from build123d import *

# Parameters (mm, degrees)
SKETCH1_R           = 1.375
BOSS_EXTRUDE1_DEPTH = 1.19
CHAMFER1_SIZE       = 0.25


with BuildPart() as part:
    # Sketch1 → Boss-Extrude1 (new, symmetric)
    with BuildSketch(Plane(origin=(0, 0, 0), x_dir=(1, 0, 0), z_dir=(0, 1, 0))):
        Polygon((0, 3.175426481), (-2.75, 1.58771324), (-2.75, -1.58771324), (0, -3.175426481), (2.75, -1.58771324), (2.75, 1.58771324), align=None)
        with Locations(Location((0, 0, 0), (0, 0, 270))):
            Circle(SKETCH1_R, mode=Mode.SUBTRACT)
    extrude(amount=BOSS_EXTRUDE1_DEPTH, both=True)

    # Sketch2 → Cut-Revolve1 (revolve, cut)
    with BuildSketch(Plane(origin=(0, 0, 0), x_dir=(0, 0, -1), z_dir=(1, 0, 0))):
        Polygon((2.7, 1.19), (3.175426481, 0.89), (3.175426481, 1.19), align=None)
    cut_revolve1 = revolve(axis=Axis((0, 0, 0), (0, 1, 0)), mode=Mode.SUBTRACT)

    # Mirror1: Cut-Revolve1 across plane
    add(cut_revolve1.mirror(Plane.ZX), mode=Mode.SUBTRACT)

    # Chamfer1
    chamfer1_edges = [part.edges().sort_by_distance(p)[0] for p in [
        (0, -1.19, -1.375),
        (0, 1.19, -1.375),
    ]]
    chamfer(chamfer1_edges, length=CHAMFER1_SIZE)


solid = part.part
For this review, take the finished solid that the model builds, in its own axes (mm). Round coordinates to 2 decimals unless told otherwise and drop trailing zeros. Write each loop counter-clockwise with the first axis right and the second up, starting at its lowest first coordinate (ties: lowest second). Pieces come first, ordered by that corner, then holes. Notation, with made-up numbers: (27.25, -1) -> (82.25, -1) arc R32 ccw to (82.25, 34) -> close; hole circle Ø7 at (14, -9.75). An arc over 180 degrees is marked (long way). Put each result on its own line as item: value.
Q1. Consider section B-B on y = 0.5. State the section outline as (x, z) points (3 decimals).
Determined:
outline: (-2.75, -1.588) -> (0, -3.175) -> (2.75, -1.588) -> (2.75, 1.588) -> (0, 3.175) -> (-2.75, 1.588) -> close; hole circle Ø2.75 at (0, 0)
Q2. Consider section A-A on z = 0. State the section outline as (x, y) points (3 decimals).
Determined:
outline: (-2.75, -1.158) -> (-2.7, -1.19) -> (-1.625, -1.19) -> (-1.375, -0.94) -> (-1.375, 0.94) -> (-1.625, 1.19) -> (-2.7, 1.19) -> (-2.75, 1.158) -> close; (1.375, -0.94) -> (1.625, -1.19) -> (2.7, -1.19) -> (2.75, -1.158) -> (2.75, 1.158) -> (2.7, 1.19) -> (1.625, 1.19) -> (1.375, 0.94) -> close
Q3. The part is to be moulded in two halves that separate along Z. For faces 1 (the cylindrical face through (-1.34, -0.01, -0.3)), 2 (the conical face through (0, -1, 3)), 3 (the flat face through (0, -1.19, 2)), say which applies: released by +Z, released by -Z, zero draft, split by the parting line, or undercut.
Determined:
face 1: undercut
face 2: split by the parting line
face 3: zero draft
Q4. To check wall thickness, follow L1, parallel to X at y = -0.2, z = 0 (3 decimals); L2, parallel to X at y = 0.6, z = 1.25; L3, parallel to Z at x = -0.6, y = -0.9. State the ranges of each line that lie inside material, in increasing order. Write a range as [from, to].
Determined:
L1: x = [-2.75, -1.375], [1.375, 2.75]
L2: x = [-2.75, -0.57], [0.57, 2.75]
L3: z = [-2.83, -1.24], [1.24, 2.83]
